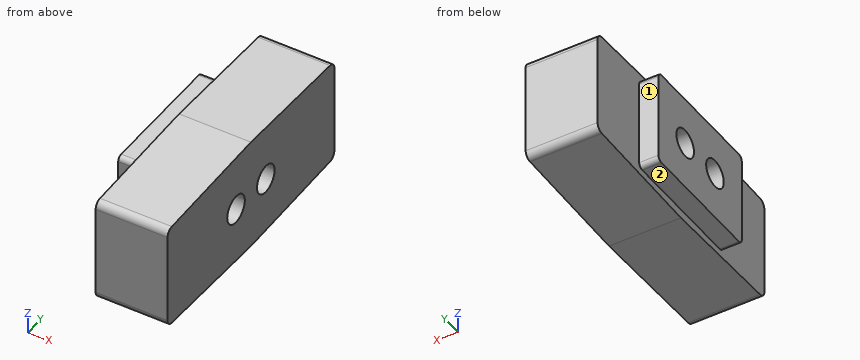
```python
from build123d import *

# Parameters (mm, degrees)
BOSS_EXTRUDE1_DEPTH     = 3.81
BOSS_EXTRUDE2_DEPTH     = 1.016
CUT_EXTRUDE1_DEPTH      = 16.636574662
CUT_EXTRUDE1_DEPTH_BACK = 16.636574662
SKETCH6_R               = 0.75


with BuildPart() as part:
    # Sketch1 → Boss-Extrude1 (new body)
    with BuildSketch(Plane(origin=(0, 0, 0), x_dir=(0, 0, -1), z_dir=(1, 0, 0))):
        with BuildLine():
            Line((0.380788543, -13.474691937), (0.605560313, -6.731))
            Line((0.605560313, -6.731), (0.380788543, 0.012691937))
            ThreePointArc((0.380788543, 0.012691937), (0.2648824, 0.273858201), (0, 0.381))
            Line((0, 0.381), (-4.833515176, 0.381))
            ThreePointArc((-4.833515176, 0.381), (-5.098397576, 0.273858201), (-5.214303719, 0.012691937))
            Line((-5.214303719, 0.012691937), (-5.439075489, -6.731))
            Line((-5.439075489, -6.731), (-5.214303719, -13.474691937))
            ThreePointArc((-5.214303719, -13.474691937), (-5.098397576, -13.735858201), (-4.833515176, -13.843))
            Line((-4.833515176, -13.843), (0, -13.843))
            ThreePointArc((0, -13.843), (0.2648824, -13.735858201), (0.380788543, -13.474691937))
        make_face()
    extrude(amount=BOSS_EXTRUDE1_DEPTH)

    # Sketch5 → Boss-Extrude2 (add)
    with BuildSketch(Plane.ZY):
        with BuildLine():
            Line((0.130757588, -10.287), (4.702757588, -10.287))
            ThreePointArc((4.702757588, -10.287), (4.88236271, -10.212605122), (4.956757588, -10.033))
            Line((4.956757588, -10.033), (4.956757588, -3.429))
            ThreePointArc((4.956757588, -3.429), (4.88236271, -3.249394878), (4.702757588, -3.175))
            Line((4.702757588, -3.175), (0.130757588, -3.175))
            ThreePointArc((0.130757588, -3.175), (-0.048847535, -3.249394878), (-0.123242412, -3.429))
            Line((-0.123242412, -3.429), (-0.123242412, -10.033))
            ThreePointArc((-0.123242412, -10.033), (-0.048847535, -10.212605122), (0.130757588, -10.287))
        make_face()
    extrude(amount=BOSS_EXTRUDE2_DEPTH)

    # Sketch6 → Cut-Extrude1 (cut, two sides: drawn at the far end of the back side and taken through both)
    with BuildSketch(Plane.ZY.offset(1.016).offset(-CUT_EXTRUDE1_DEPTH_BACK)):
        with Locations((2.416757588, -5.461)):
            Circle(SKETCH6_R)
        with Locations((2.416757588, -8.001)):
            Circle(SKETCH6_R)
    extrude(amount=CUT_EXTRUDE1_DEPTH + CUT_EXTRUDE1_DEPTH_BACK, mode=Mode.SUBTRACT)


solid = part.part
```
Here's how the part is built. I have some questions about the finished solid (model axes, mm). Face numbers are marked on the shaded views. Coordinates: 2 decimals unless noted, no trailing zeros. Loops run counter-clockwise (first coordinate to the right, second up) from the corner with the lowest first, then second, coordinate; pieces in that order, holes last. Notation, with made-up numbers: (36, 17) - (80, 17) arc R32 ccw to (80, 55) - close; hole circle Ø11 at (-35.5, 5). An arc over 180 degrees is marked (long way). Return JSON: item names as keys, results as strings. Group by question number.
Item 1: If we section it at D-D on z = 2.5: Write out the boundary of the cut face in (x, y) (3 decimals), and give its area (3 significant figures).
Item 2: If we section it at B-B on x = 2.75: Write out the boundary of the cut face in (y, z), and give its area (3 significant figures).
Item 3: We'd pull the mould along Z, two halves only. Please class the marked faces 1 and 2: +Z half, -Z half, draft (parallel to the pull), parting line (faces both ways), or undercut.
Item 4: If we section it at A-A on z = 0.75: Write out the boundary of the cut face in (x, y) (3 decimals), and give its area (3 significant figures).
Item 5: Will these pins go through, and if not, where does the flat tip stop? P1, Ø0.5, axis at x = -0.5, y = -5.5, coming from the +Z side; P2, Ø0.5, axis at x = -0.5, z = 2, coming from the -Y side; P3, Ø1.5, axis at x = 1.5, y = -6.5, coming from the +Z side; P4, Ø1.2, axis at y = -8, z = 2.42, coming from the -X side.
Item 6: I need wall thicknesses on line 1 (Y direction, x = 0.65, z = 2.75); line 2 (Y direction, x = -0.65, z = 3.75) (3 decimals); line 3 (Z direction, x = -0.55, y = -4). Which ranges of each line are inside material? Lowest first, please. Write a range as from..to.
Item 7: If we section it at C-C on y = -5: Write out the boundary of the cut face in (x, z), and give its area (3 significant figures).
Calculated:
{
 "1": {"outline": "(-1.016, -10.287) - (0, -10.287) - (0, -13.843) - (3.81, -13.843) - (3.81, -8.746) - (-1.016, -8.746) - close; (-1.016, -7.256) - (3.81, -7.256) - (3.81, -6.206) - (-1.016, -6.206) - close; (-1.016, -4.716) - (3.81, -4.716) - (3.81, 0.381) - (0, 0.381) - (0, -3.175) - (-1.016, -3.175) - close", "area": "47.0 mm^2"},
 "2": {"outline": "(-13.84, 0) arc R0.38 ccw to (-13.47, -0.38) - (-6.73, -0.61) - (0.01, -0.38) arc R0.38 ccw to (0.38, 0) - (0.38, 4.83) arc R0.38 ccw to (0.01, 5.21) - (-6.73, 5.44) - (-13.47, 5.21) arc R0.38 ccw to (-13.84, 4.83) - close; hole circle Ø1.5 at (-8, 2.42); hole circle Ø1.5 at (-5.46, 2.42)", "area": "79.0 mm^2"},
 "3": {"face 1": "draft", "face 2": "-Z half"},
 "4": {"outline": "(-1.016, -10.287) - (0, -10.287) - (0, -13.843) - (3.81, -13.843) - (3.81, 0.381) - (0, 0.381) - (0, -3.175) - (-1.016, -3.175) - close", "area": "61.4 mm^2"},
 "5": {"P1": "stops at z = 4.96", "P2": "stops at y = -10.29", "P3": "stops at z = 5.44", "P4": "passes through"},
 "6": {"line 1": "y = -13.84..-8.67, -7.33..-6.13, -4.79..0.38", "line 2": "y = -10.287..-3.175", "line 3": "z = -0.12..4.96"},
 "7": {"outline": "(-1.02, -0.12) - (0, -0.12) - (0, -0.55) - (3.81, -0.55) - (3.81, 1.83) - (-1.02, 1.83) - close; (-1.02, 3.01) - (3.81, 3.01) - (3.81, 5.38) - (0, 5.38) - (0, 4.96) - (-1.02, 4.96) - close", "area": "22.0 mm^2"}
}
